Read the model definition and answer for the solid it produces. Units are mm, in the model's axes. A direction names the side the tool comes from. Coordinates: 2 decimals unless noted, no trailing zeros. Order: outer loops, then holes, each group sorted by start corner. A loop starts at its lowest first (then second) coordinate and runs counter-clockwise, first axis right, second up.
from build123d import *


# Read off the part's stored shape, not the designer's step: 1/4 NPT Tapped Hole1
with BuildPart() as part:
    # Sketch1 → Revolve1 (revolve)
    with BuildSketch(Plane.XY, mode=Mode.PRIVATE) as revolve1_sk:
        Polygon((-17.78, 0), (-17.78, 30), (-30.48, 30), (-30.48, 4), (-43.18, 4), (-43.18, 0), align=None)
    revolve(revolve1_sk.sketch.rotate(Axis((0, 0, 0), (0, 1, 0)), 270), axis=Axis((0, 0, 0), (0, 1, 0)))

    # 1/4 NPT Tapped Hole1 outline → 1/4 NPT Tapped Hole1 (revolve, cut)
    with BuildSketch(Plane.XZ.offset(-13.590721134)):
        Polygon((5.5626, 20.46), (5.943676082, 20.46), (6.243695498, 30.480240418), (0, 30.480240418), (0, 16.886929185), (5.5626, 16.886929185), align=None)
    revolve(axis=Axis((0, 13.590721134, 0), (0, 0, 1)), mode=Mode.SUBTRACT)


solid = part.part
Q1. Each of these flat-tipped pins is pushed along its axis until it touches: P1, Ø9.5, axis at x = 3, y = 15, coming from the +Z side; P2, Ø10, axis at x = 0, y = 13.59, coming from the -Z side; P3, Ø3, axis at y = 21, z = 21.5, coming from the +X side. Where does it stop, or does it pass through?
Q2. The part is cut by section C-C, the plane y = 2. Determine the outline of the cut face in (x, z), then the cut area to 3 significant figures.
Q3. Determine the mould class of faces 4 (the conical face through (-6.09, 13.86, 25.54)), 5 (the cylindrical face through (-29.18, 1.97, 31.83)), 6 (the flat face through (13, 30, 13)) for opening direction X: +X half, -X half, draft (parallel to the pull), parting line (faces both ways), or undercut.
Q4. The part is cut by section D-D, the plane z = 23.5. Determine the outline of the cut face in (x, y), then the cut area to 3 significant figures.
Q5. Which of the six approach directions +Z, -Z, +X, -X, +Y, -Y give full straight-line access (tool end or side, diameter ignored) to faces 1 (the flat face through (-2.2, 8.3, 20.46)), 2 (the cylindrical face through (6.81, 15.21, -16.424)), 3 (the cylindrical face through (-9.16, 16.82, -29.07))?
Q6. Straight lines are drawn through the part: L1, parallel to X at y = 6.5, z = -0.5; L2, parallel to Y at x = 0, z = 18; L3, parallel to Y at x = 31, z = -24.5. For each, find the intervals that lie inside material, in ascending order.
Q7. The part is cut by section B-B, the plane z = 0. Determine the outline of the cut face in (x, y).
Q8. The part is cut by section A-A, the plane x = 0. Determine the outline of the cut face in (y, z), then the cut area to 3 significant figures.
Computed values:
1. P1: stops at z = 30.43
1. P2: stops at z = -30.48
1. P3: stops at x = 23
2. outline: circle Ø86.36 at (0, 0); hole circle Ø35.56 at (0, 0)
2. area: 4,860 mm2
3. face 4: undercut
3. face 5: parting line
3. face 6: draft
4. outline: (-36.23, 0) - (36.23, 0) - (36.23, 4) - (19.41, 4) - (19.41, 30) - (-19.41, 30) - (-19.41, 4) - (-36.23, 4) - close; hole circle Ø12.07 at (0, 13.59)
4. area: 1,180 mm2
5. face 1: +Z
5. face 2: +Y, -Y
5. face 3: +Y
6. L1: x = -30.48 to -17.77, 17.77 to 30.48
6. L2: y = 0 to 8.03, 19.15 to 30
6. L3: y = 0 to 4
7. outline: (-43.18, 0) - (-17.78, 0) - (-17.78, 30) - (-30.48, 30) - (-30.48, 4) - (-43.18, 4) - close; (17.78, 0) - (43.18, 0) - (43.18, 4) - (30.48, 4) - (30.48, 30) - (17.78, 30) - close
8. outline: (0, -43.18) - (4, -43.18) - (4, -30.48) - (30, -30.48) - (30, -17.78) - (0, -17.78) - close; (0, 17.78) - (8.03, 17.78) - (8.03, 20.46) - (7.65, 20.46) - (7.35, 30.48) - (4, 30.48) - (4, 43.18) - (0, 43.18) - close; (19.15, 17.78) - (30, 17.78) - (30, 30.48) - (19.83, 30.48) - (19.53, 20.46) - (19.15, 20.46) - close
8. area: 712 mm2
